Verification items for the finished model (mm, model axes). A direction names the side the tool comes from. Coordinates: 2 decimals unless noted, no trailing zeros. Order: outer loops, then holes, each group sorted by start corner. A loop starts at its lowest first (then second) coordinate and runs counter-clockwise, first axis right, second up.
Q1. Thickness scan on line 1 (X direction, y = 49, z = 4.5); line 2 (Y direction, x = 93.5, z = 3.25); line 3 (Y direction, x = 109.5, z = 2.5). Record the ranges inside material, lowest first.
Q2. Cross-section at B-B, the plane z = 3.75. Record the boundary of the cut face in (x, y), and give its area (3 significant figures).
Q3. Depth check by flat-ended pin: P1, Ø1.5, axis at y = 66.5, z = 1, coming from the +X side; P2, Ø5, axis at y = 59, z = 5.5, coming from the -X side; P3, Ø5, axis at x = 126, z = 2.5, coming from the +Y side. Enter the tip coordinate at first touch or a pass-through.
Q4. Cross-section at D-D, the plane x = 97.5. Record the boundary of the cut face in (y, z), and give its area (3 significant figures).
Q5. Draft check along Y on faces 4 (the flat face through (109, 37.138, 5)), 5 (the flat face through (109, 50, 0)), 6 (the flat face through (123, 43.138, 5)), 7 (the cylindrical face through (113.14, 55.22, 4.93)). Enter one of: pulls with the +Y half, pulls with the -Y half, needs draft (parallel to the pull), parting line crosses it, or undercut.
Q6. Cross-section at A-A, the plane y = 53.5. Record the boundary of the cut face in (x, z), and give its area (3 significant figures).
Q7. Cross-section at C-C, the plane x = 107. Record the boundary of the cut face in (y, z).
Q8. Set-up check for faces 1 (the flat face through (117.523, 57, 5)), 2 (the flat face through (108, 70.138, 5)), 3 (the flat face through (99.523, 56, 5)): record each of +Z, -Z, +X, -X, +Y, -Y from which the full face is reachable in a straight line by a thin tool's end or side.
from build123d import *

# Parameters (mm, degrees)
SKETCH_R      = 5
EXTRUDE_DEPTH = 10


with BuildPart() as part:
    # Sketch → Extrude (new body)
    with BuildSketch(Plane.XY):
        Polygon((28.522638, 37.138413), (28.522638, 43.138413), (40.522638, 43.138413), (40.522638, 70.138413), (58.522638, 70.138413), (58.522638, 43.138413), (70.522638, 43.138413), (70.522638, 37.138413), align=None)
        with Locations((49.522638, 57.138413)):
            Circle(SKETCH_R, mode=Mode.SUBTRACT)
    extrude(amount=EXTRUDE_DEPTH)


with BuildPart() as part_1:
    # Extrude placement: moved
    add(part.part.moved(Location((59, 0, 0))))


solid = part_1.part
Check values:
1. line 1: x = 99.52 to 117.52
1. line 2: y = 37.14 to 43.14
1. line 3: y = 37.14 to 52.23, 62.04 to 70.14
2. outline: (87.52, 37.14) - (129.52, 37.14) - (129.52, 43.14) - (117.52, 43.14) - (117.52, 70.14) - (99.52, 70.14) - (99.52, 43.14) - (87.52, 43.14) - close; hole circle Ø10 at (108.52, 57.14)
2. area: 659 mm2
3. P1: stops at x = 117.52
3. P2: stops at x = 99.52
3. P3: stops at y = 43.14
4. outline: (37.14, 0) - (43.14, 0) - (43.14, 10) - (37.14, 10) - close
4. area: 60.0 mm2
5. face 4: pulls with the -Y half
5. face 5: needs draft
5. face 6: pulls with the +Y half
5. face 7: undercut
6. outline: (99.52, 0) - (105.09, 0) - (105.09, 10) - (99.52, 10) - close; (111.95, 0) - (117.52, 0) - (117.52, 10) - (111.95, 10) - close
6. area: 111 mm2
7. outline: (37.14, 0) - (52.38, 0) - (52.38, 10) - (37.14, 10) - close; (61.9, 0) - (70.14, 0) - (70.14, 10) - (61.9, 10) - close
8. face 1: +Z, -Z, +X, +Y
8. face 2: +Z, -Z, +X, -X, +Y
8. face 3: +Z, -Z, -X, +Y
